Study the drawing (mm; zero at the part's minimum x, y, z) and answer. A direction names the side the tool comes from. Coordinates: 2 decimals unless noted, no trailing zeros. Loops run counter-clockwise (first coordinate to the right, second up) from the corner with the lowest first, then second, coordinate; pieces in that order, holes last. Notation, with made-up numbers: (81, 58) - (93, 58) arc R21 ccw to (93, 96) - close; hole circle Ø9 at (85.25, 34). An arc over 180 degrees is marked (long way). Use one line per item in the form item = value.
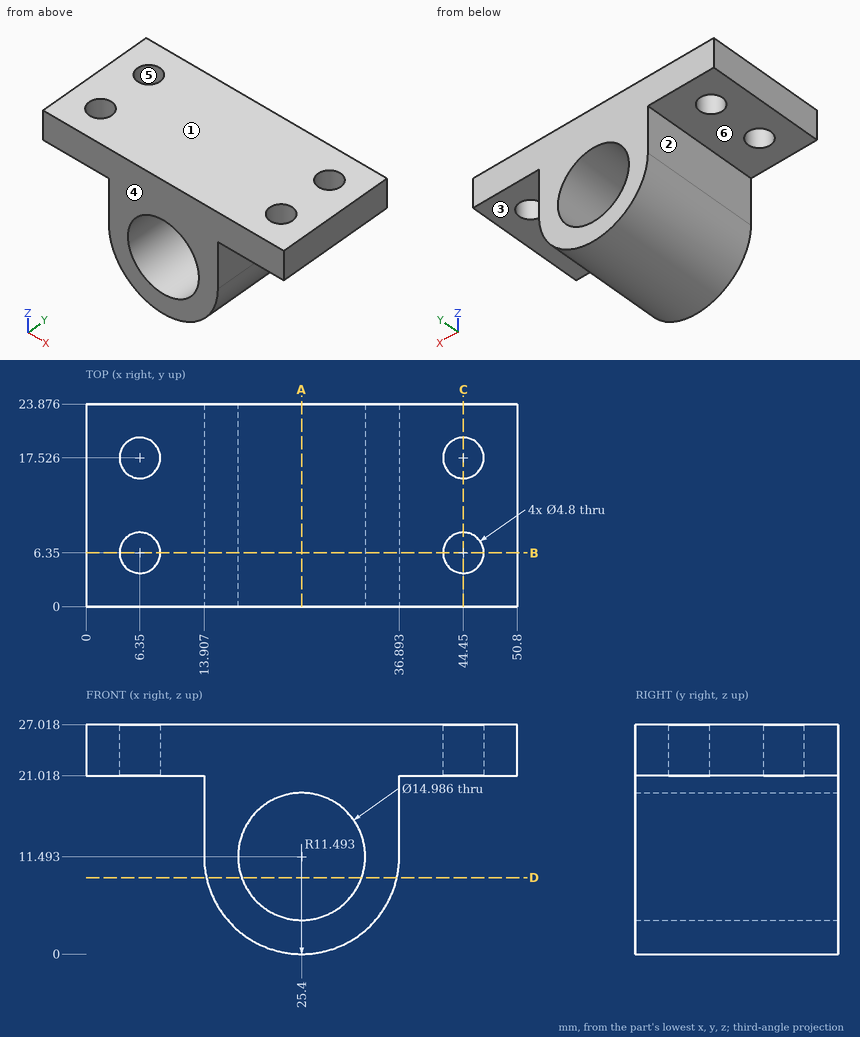
Item 1: For a pull along Y with two mould halves and no side action, classify the marked faces 4, 5 and 6 as +Y half, -Y half, draft (parallel to the pull), parting line (faces both ways), or undercut.
Results below:
face_4 = -Y half
face_5 = undercut
face_6 = draft
Item 2: Find the intervals of material crossed by L1, parallel to Y at x = 44.45, z = 23.3; L2, parallel to Z at x = 8, y = 19.75; L3, parallel to Z at x = 25.4, y = 18, in increasing order.
Results below:
L1 = 0 to 3.95, 8.75 to 15.13, 19.93 to 23.88
L2 = 21.02 to 27.02
L3 = 0 to 4, 18.99 to 27.02
Item 3: The part is cut by section A-A on x = 25.4. Give the vertices of the cut face in (y, z).
Results below:
outline = (0, 0) - (23.88, 0) - (23.88, 4) - (0, 4) - close; (0, 18.99) - (23.88, 18.99) - (23.88, 27.02) - (0, 27.02) - close
Item 4: The part is cut by section C-C on x = 44.45. Give the vertices of the cut face in (y, z).
Results below:
outline = (0, 21.02) - (3.95, 21.02) - (3.95, 27.02) - (0, 27.02) - close; (8.75, 21.02) - (15.13, 21.02) - (15.13, 27.02) - (8.75, 27.02) - close; (19.93, 21.02) - (23.88, 21.02) - (23.88, 27.02) - (19.93, 27.02) - close
Item 5: Each of these flat-tipped pins is pushed along its axis until it touches: P1, Ø12, axis at y = 9.5, z = 10, coming from the +X side; P2, Ø11, axis at x = 45, y = 10, coming from the -Z side; P3, Ø10, axis at y = 4, z = 17, coming from the -X side; P4, Ø1, axis at y = 8.5, z = 5, coming from the -X side. Where does it stop, or does it pass through?
Results below:
P1 = 36.89
P2 = 21.02
P3 = 0
P4 = 15.59
Item 6: The part is cut by section B-B on y = 6.35. Give the vertices of the cut face in (x, z), plus the area to 3 significant figures.
Results below:
outline = (0, 21.02) - (3.95, 21.02) - (3.95, 27.02) - (0, 27.02) - close; (8.75, 21.02) - (13.91, 21.02) - (13.91, 11.49) arc R11.49 ccw to (36.89, 11.49) - (36.89, 21.02) - (42.05, 21.02) - (42.05, 27.02) - (8.75, 27.02) - close; (46.85, 21.02) - (50.8, 21.02) - (50.8, 27.02) - (46.85, 27.02) - close; hole circle Ø14.99 at (25.4, 11.49)
area = 497 mm²
Item 7: The part is cut by section D-D on z = 9. Give the vertices of the cut face in (x, y).
Results below:
outline = (14.18, 0) - (18.33, 0) - (18.33, 23.88) - (14.18, 23.88) - close; (32.47, 0) - (36.62, 0) - (36.62, 23.88) - (32.47, 23.88) - close
Item 8: Which of the six approach directions +Z, -Z, +X, -X, +Y, -Y give full straight-line access (tool end or side, diameter ignored) to the marked faces 1, 2 and 3?
Results below:
face_1 = +Z, +X, -X, +Y, -Y
face_2 = -Z, -X, +Y, -Y
face_3 = -Z, +X, +Y, -Y
